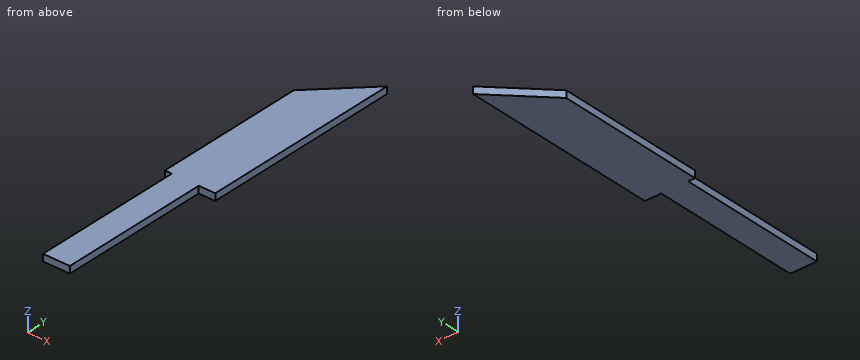
Autodesk Inventor part; units mm, degrees
ref_plane "YZ Plane" through (0, 0, 0) normal (1, 0, 0) x (0, 1, 0)
ref_plane "XZ Plane" through (0, 0, 0) normal (0, 1, 0) x (-1, 0, 0)
ref_plane "XY Plane" through (0, 0, 0) normal (0, 0, 1) x (1, 0, 0)
sketch "Sketch1" plane through (0, 0, 0) normal (0, 0, 1) x (1, 0, 0)
  line L0 (-10, 0) -> (-10, 10)
  line L1 (0, 10) -> (0, 0)
  line L2 (-8.623, 0) -> (-8.623, -30)
  line L3 (-8.623, -30) -> (-3.288, -30)
  line L4 (-3.288, -30) -> (-3.288, 0)
  line L5 (0, 40) -> (-10, 30)
  line L6 (0, 40) -> (14.1421, 40) construction
  line L7 (-10, 30) -> (-10, 10)
  line L8 (-3.288, 0) -> (0, 0)
  line L9 (-8.623, 0) -> (-10, 0)
  line L10 (0, 40) -> (0, 10)
  dimension "d0" = 10
  dimension "d1" = 10
  dimension "d2" = 5.335
  dimension "d3" = 30
  dimension "d4" = 3.288
  dimension "d5" = 1.377
  dimension "d7" = 135
extrude "Extrusion1" add sketch "Sketch1" along normal blind 1.375
properties part number "bladex1"
Input: part model. Units: mm. Frame: model coordinates. Coordinates: 2 decimals unless noted, no trailing zeros. Loops run counter-clockwise (first coordinate to the right, second up) from the corner with the lowest first, then second, coordinate; pieces in that order, holes last. Notation, with made-up numbers: (24.5, 46.5) -> (30.5, 46.5) arc R14 cw to (30.5, 61.5) -> close; hole circle Ø10 at (67, -30.75). An arc over 180 degrees is marked (long way). Use a Markdown table: item, result.
1) Material intervals for line 1 along X through (y, z) = (-25, 0.85); line 2 along Y through (x, z) = (-7.75, 0.15); line 3 along Y through (x, z) = (-4.5, 0.5), sorted ascending. Write a range as from..to.
Results found:
| item | result |
|---|---|
| line 1 | x = -8.62..-3.29 |
| line 2 | y = -30..32.25 |
| line 3 | y = -30..35.5 |
2) Cut plane C-C (x = -4). Return the cut outline in (y, z) (3 decimals), then the cut area to 4 significant figures.
Results found:
| item | result |
|---|---|
| outline | (-30, 0) -> (36, 0) -> (36, 1.375) -> (-30, 1.375) -> close |
| area | 90.75 mm2 |
3) Cut plane A-A (z = 0.4). Return the cut outline in (x, y).
Results found:
| item | result |
|---|---|
| outline | (-10, 0) -> (-8.62, 0) -> (-8.62, -30) -> (-3.29, -30) -> (-3.29, 0) -> (0, 0) -> (0, 40) -> (-10, 30) -> close |
4) Contact query for a flat-ended pin moving along its axis: pin 1 (0.7 mm diameter, centred on y = -10, z = 0.5, fed in from +X). Output: stop coordinate, or through.
Results found:
| item | result |
|---|---|
| pin 1 | stops at x = -3.29 |
5) Cut plane B-B (y = 33). Return the cut outline in (x, z) (3 decimals), then the cut area to 4 significant figures.
Results found:
| item | result |
|---|---|
| outline | (-7, 0) -> (0, 0) -> (0, 1.375) -> (-7, 1.375) -> close |
| area | 9.625 mm2 |
